Autodesk Inventor part; units mm, degrees
ref_plane "YZ Plane" through (0, 0, 0) normal (1, 0, 0) x (0, 1, 0)
ref_plane "XZ Plane" through (0, 0, 0) normal (0, 1, 0) x (-1, 0, 0)
ref_plane "XY Plane" through (0, 0, 0) normal (0, 0, 1) x (1, 0, 0)
sketch "Sketch1" plane through (0, 0, 0) normal (1, 0, 0) x (0, 1, 0)
  line L0 (-116.4234, 72.9982) -> (-116.4234, -7.0018)
  line L1 (-111.4234, -12.0018) -> (-86.4234, -12.0018)
  line L2 (-81.4234, -7.0018) -> (-81.4234, 72.9982)
  line L3 (-90.9234, 75.9982) -> (-90.9234, 55.9982)
  line L4 (-92.9234, 53.9982) -> (-104.9234, 53.9982)
  line L5 (-106.9234, 55.9982) -> (-106.9234, 75.9982)
  line L6 (-86.4234, 77.9982) -> (-88.9234, 77.9982)
  line L7 (-108.9234, 77.9982) -> (-111.4234, 77.9982)
  circle A0 centre (-98.1419, 27.9982) radius 7.5
  circle A1 centre (-98.1419, 2.9982) radius 5.1
  circle A2 centre (-110.1419, 27.9982) radius 2
  circle A3 centre (-112.4234, 61.8916) radius 2
  circle A4 centre (-56.4234, 61.8916) radius 2
  circle A5 centre (-106.1419, 2.9982) radius 2
  circle A6 centre (-98.1419, 15.9982) radius 2
  circle A7 centre (-86.1419, 27.9982) radius 2
  circle A8 centre (-98.1419, 39.9982) radius 2
  circle A9 centre (-98.1419, -5.0018) radius 2
  circle A10 centre (-90.1419, 2.9982) radius 2
  circle A11 centre (-98.1419, 10.9982) radius 2
  arc A12 (-111.4234, 77.9982) -> (-116.4234, 72.9982) centre (-111.4234, 72.9982) ccw
  arc A13 (-81.4234, 72.9982) -> (-86.4234, 77.9982) centre (-86.4234, 72.9982) ccw
  arc A14 (-116.4234, -7.0018) -> (-111.4234, -12.0018) centre (-111.4234, -7.0018) ccw
  arc A15 (-86.4234, -12.0018) -> (-81.4234, -7.0018) centre (-86.4234, -7.0018) ccw
  arc A16 (-106.9234, 55.9982) -> (-104.9234, 53.9982) centre (-104.9234, 55.9982) ccw
  arc A17 (-92.9234, 53.9982) -> (-90.9234, 55.9982) centre (-92.9234, 55.9982) ccw
  arc A18 (-106.9234, 75.9982) -> (-108.9234, 77.9982) centre (-108.9234, 75.9982) ccw
  arc A19 (-88.9234, 77.9982) -> (-90.9234, 75.9982) centre (-88.9234, 75.9982) ccw
  point P0 (-81.4234, 77.9982)
  point P1 (-116.4234, -12.0018)
  point P2 (-116.4234, 77.9982)
  point P3 (-81.4234, -12.0018)
  point P4 (-90.9234, 77.9982)
  point P5 (-90.9234, 53.9982)
  point P6 (-106.9234, 53.9982)
  point P7 (-106.9234, 77.9982)
  dimension "d29" = 360
  dimension "d44" = 35
  dimension "d45" = 90
  dimension "d46" = 16
  dimension "d47" = 24
  dimension "d48" = 15
  dimension "d53" = 10.2
  dimension "d54" = 25
  dimension "d55" = 26
  dimension "d58" = 56
  dimension "d59" = 4
  dimension "d60" = 4
  dimension "d62" = 12
  dimension "d63" = 8
  dimension "d66" = 360
  dimension "d70" = 360
  dimension "d72" = 5
  dimension "d73" = 2
extrude "Extrusion1" add sketch "Sketch1" along normal blind 6.35 contours A12 L7 A18 L5 A16 L4 A17 L3 A19 L6 A13 L2 A15 L1 A14 L0 | A3 | A6 | A11
properties part number "carriage"
Part model, mm, in its own coordinate system. A direction names the side the tool comes from. Round coordinates to 2 decimals unless told otherwise and drop trailing zeros. Order: outer loops, then holes, each group sorted by start corner. A loop starts at its lowest first (then second) coordinate and runs counter-clockwise, first axis right, second up. Notation, with made-up numbers: M 1.25,53 L 26.25,53 A9 ccw 26.25,67 Z; hole C 51,-18.75 d9. An arc over 180 degrees is marked long. Answer in a Markdown table with one row per item. Add a question column.
Q1. Pin check, flat tips, straight feed: pin 1 (1.9 mm diameter, centred on x = 4.5, y = -97, fed in from +Z); pin 2 (5 mm diameter, centred on y = -110.14, z = 28, fed in from -X); pin 3 (3 mm diameter, centred on y = -98.14, z = 40, fed in from -X); pin 4 (2 mm diameter, centred on x = 1, y = -92.5, fed in from +Z). Stop position of each tip, or through.
Q2. Mould opens along Y. For faces 1 (the face through (0, -107, 34)), 2 (the face through (3.131, -82.927, 76.572)), 3 (the face through (3.13, -92.14, 2.91)) say: +Y half, -Y half, draft (parallel to the pull), parting line (faces both ways), or undercut.
Q3. Cut at A-A on z = 70. Give the cut face in (x, y), and give its area (3 significant figures).
Q4. Cut at D-D on x = 4.25. Give the number of separate pieces and of enclosed holes in the cut face, and give its area (3 significant figures).
Q5. 3-axis set-ups, long thin cutter, end or side, ignore diameter. For faces 4 (the face through (3, -90.923, 66)), 5 (the face through (3.131, -109.219, 29.773)): which of +Z, -Z, +X, -X, +Y, -Y reach the whole face in a straight line?
Q6. Cut at B-B on z = 27. Give the cut face in (x, y), and give its area (3 significant figures).
Q7. Cut at C-C on y = -94.5. Give the cut face in (x, z).
Q8. Wall check: L1, parallel to Z at x = 4, y = -98; L2, parallel to Y at x = 5, z = 68; L3, parallel to Z at x = 5.25, y = -99.5. Give the ranges that are in metal, low to high. Write a range as from..to.
Established:
| question | item | result |
|---|---|---|
| 1 | pin 1 | stops at z = 54 |
| 1 | pin 2 | stops at x = 0 |
| 1 | pin 3 | passes through |
| 1 | pin 4 | stops at z = 54.59 |
| 2 | face 1 | draft |
| 2 | face 2 | +Y half |
| 2 | face 3 | undercut |
| 3 | outline | M 0,-116.42 L 6.35,-116.42 L 6.35,-106.92 L 0,-106.92 Z; M 0,-90.92 L 6.35,-90.92 L 6.35,-81.42 L 0,-81.42 Z |
| 3 | area | 121 mm2 |
| 4 | separate pieces | 1 |
| 4 | enclosed holes | 8 |
| 4 | area | 2,410 mm2 |
| 5 | face 4 | +Z, +X, -X |
| 5 | face 5 | +X, -X |
| 6 | outline | M 0,-116.42 L 6.35,-116.42 L 6.35,-111.87 L 0,-111.87 Z; M 0,-108.41 L 6.35,-108.41 L 6.35,-105.58 L 0,-105.58 Z; M 0,-90.71 L 6.35,-90.71 L 6.35,-87.87 L 0,-87.87 Z; M 0,-84.41 L 6.35,-84.41 L 6.35,-81.42 L 0,-81.42 Z |
| 6 | area | 83.8 mm2 |
| 7 | outline | M 0,-12 L 6.35,-12 L 6.35,-0.57 L 0,-0.57 Z; M 0,6.57 L 6.35,6.57 L 6.35,21.44 L 0,21.44 Z; M 0,34.55 L 6.35,34.55 L 6.35,54 L 0,54 Z |
| 8 | L1 | z = -12..-7, -3.01..-2.1, 8.1..20.5, 35.5..38, 41.99..54 |
| 8 | L2 | y = -116.42..-106.92, -90.92..-81.42 |
| 8 | L3 | z = -12..-6.47, -3.53..-1.92, 7.91..20.62, 35.37..38.53, 41.47..54 |
